```python
from build123d import *

# Parameters (mm, degrees)
BOSS_EXTRUDE1_DEPTH = 130
FILLET1_R           = 50


with BuildPart() as part:
    # Sketch1 → Boss-Extrude1 (new body)
    with BuildSketch(Plane.XY):
        Polygon((0, 0), (58, 0), (30, -5), (0, -5), align=None)
    extrude(amount=BOSS_EXTRUDE1_DEPTH)

    # Fillet1
    fillet1_edges = [part.edges().sort_by_distance(p)[0] for p in [
        (30, -5, 65),
    ]]
    fillet(fillet1_edges, radius=FILLET1_R)


solid = part.part
```
Can you work these out from the model? Positions are in its coordinate system, mm. Give positions to 0.01 mm unless a question says otherwise; leave off trailing zeros. Order: outer loops, then holes, each group sorted by start corner. A loop starts at its lowest first (then second) coordinate and runs counter-clockwise, first axis right, second up. Notation, with made-up numbers: (77, 79.5) - (114, 79.5) arc R15 ccw to (114, 103.5) - close; hole circle Ø1 at (86, 86.25). An arc over 180 degrees is marked (long way). Use a Markdown table: item, result. Add a question column.
Q1. Please list where these lines run through material, in increasing order: line 1 along Y through (x, z) = (27, 111); line 2 along Y through (x, z) = (41, 34).
Q2. I'm going to push flat-ended pins straight in: pin 1 (12 mm diameter, centred on x = 47, z = 110.5, fed in from -Y); pin 2 (1 mm diameter, centred on x = 30.5, z = 56.5, fed in from -Y). Where does each tip first touch, or does it pass through?
Q3. If we section it at B-B on y = -2.6: Write out the boundary of the cut face in (x, z).
Q4. If we section it at A-A on z = 109.5: Write out the boundary of the cut face in (x, y), plus the area to 3 significant figures.
Q5. If we section it at C-C on x = 46.5: Write out the boundary of the cut face in (y, z), plus the area to 3 significant figures.
Answers follow:
| question | item | result |
|---|---|---|
| 1 | line 1 | y = -4.98 to 0 |
| 1 | line 2 | y = -3.04 to 0 |
| 2 | pin 1 | stops at y = -3.04 |
| 2 | pin 2 | stops at y = -4.8 |
| 3 | outline | (0, 0) - (43.44, 0) - (43.44, 130) - (0, 130) - close |
| 4 | outline | (0, -5) - (25.57, -5) arc R50 ccw to (34.36, -4.22) - (58, 0) - (0, 0) - close |
| 4 | area | 219 mm^2 |
| 5 | outline | (-2.05, 0) - (0, 0) - (0, 130) - (-2.05, 130) - close |
| 5 | area | 267 mm^2 |
